from build123d import *

# Parameters (mm, degrees)
F1_DEPTH = 25
F0_R     = 250
F2_DEPTH = 20
F0_R_2   = 130
F3_DEPTH = 15


with BuildPart() as f1:
    # F0 (on Front) → F1 (new body)
    with BuildSketch(Plane.XZ):
        with BuildLine():
            ThreePointArc((79.802773, 564.385965), (0, 490), (-79.802773, 564.385965))
            ThreePointArc((-79.802773, 564.385965), (-570, 0), (-79.802773, -564.385965))
            ThreePointArc((-79.802773, -564.385965), (0, -490), (79.802773, -564.385965))
            ThreePointArc((79.802773, -564.385965), (570, 0), (79.802773, 564.385965))
        make_face()
        with BuildLine():
            ThreePointArc((-330.670307, 225.071429), (-335.875721, 335.875721), (-225.071429, 330.670307))
            ThreePointArc((-225.071429, 330.670307), (0, 400), (225.071429, 330.670307))
            ThreePointArc((225.071429, 330.670307), (308.260755, 353.404197), (357.842712, 282.842712))
            ThreePointArc((357.842712, 282.842712), (350.710487, 250.921478), (330.670307, 225.071429))
            ThreePointArc((330.670307, 225.071429), (400, 0), (330.670307, -225.071429))
            ThreePointArc((330.670307, -225.071429), (350.710487, -250.921478), (357.842712, -282.842712))
            ThreePointArc((357.842712, -282.842712), (308.260755, -353.404197), (225.071429, -330.670307))
            ThreePointArc((225.071429, -330.670307), (0, -400), (-225.071429, -330.670307))
            ThreePointArc((-225.071429, -330.670307), (-335.875721, -335.875721), (-330.670307, -225.071429))
            ThreePointArc((-330.670307, -225.071429), (-400, 0), (-330.670307, 225.071429))
        make_face(mode=Mode.SUBTRACT)
    extrude(amount=F1_DEPTH)

    # F0 (on Front) → F2 (join)
    with BuildSketch(Plane.XZ):
        with BuildLine():
            ThreePointArc((-225.071429, 330.670307), (-212.281228, 308.260755), (-207.842712, 282.842712))
            ThreePointArc((-207.842712, 282.842712), (-250.921478, 214.974938), (-330.670307, 225.071429))
            ThreePointArc((-330.670307, 225.071429), (-400, 0), (-330.670307, -225.071429))
            ThreePointArc((-330.670307, -225.071429), (-250.921478, -214.974938), (-207.842712, -282.842712))
            ThreePointArc((-207.842712, -282.842712), (-212.281228, -308.260755), (-225.071429, -330.670307))
            ThreePointArc((-225.071429, -330.670307), (0, -400), (225.071429, -330.670307))
            ThreePointArc((225.071429, -330.670307), (229.809704, -229.809704), (330.670307, -225.071429))
            ThreePointArc((330.670307, -225.071429), (400, 0), (330.670307, 225.071429))
            ThreePointArc((330.670307, 225.071429), (229.809704, 229.809704), (225.071429, 330.670307))
            ThreePointArc((225.071429, 330.670307), (0, 400), (-225.071429, 330.670307))
        make_face()
        Circle(F0_R, mode=Mode.SUBTRACT)
    extrude(amount=F2_DEPTH)

    # F0 (on Front) → F3 (join)
    with BuildSketch(Plane.XZ):
        Circle(F0_R)
        Circle(F0_R_2, mode=Mode.SUBTRACT)
    extrude(amount=F3_DEPTH)


solid = f1.part
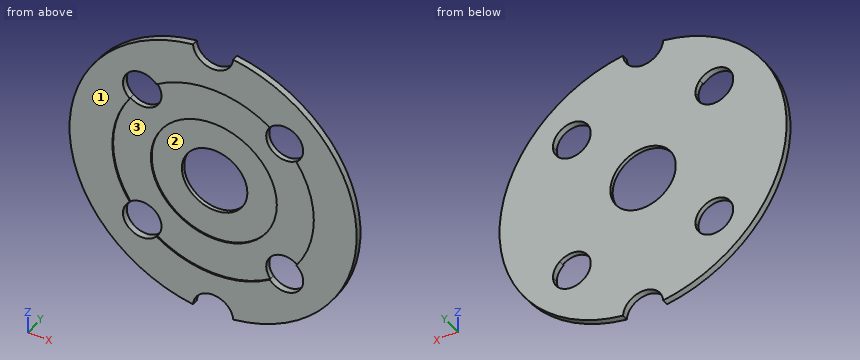
Build history of the part. All positions in model axes, mm. Face numbers are marked on the shaded views. Round coordinates to 2 decimals unless told otherwise and drop trailing zeros. Write each loop counter-clockwise with the first axis right and the second up, starting at its lowest first coordinate (ties: lowest second). Pieces come first, ordered by that corner, then holes. Notation, with made-up numbers: (31.5, 55.25) -> (37.5, 55.25) arc R33 ccw to (37.5, 88.25) -> close; hole circle Ø2 at (16.25, -2). An arc over 180 degrees is marked (long way). Use one line per item in the form item = value.
Q1. Drop flat-ended pins along their axis: P1, Ø1, axis at x = 405.5, y = -18.5, coming from the -Z side; P2, Ø8, axis at x = 175.5, z = 79, coming from the -Y side; P3, Ø2, axis at x = -321, y = -20.5, coming from the -Z side. Give the stop position or say it passes through.
Conclusion:
P1 = -401.09
P2 = -15
P3 = -471.7
Q2. Band-saw the part on B-B, the plane x = 313. Write the cut outline in (y, z).
Conclusion:
outline = (-25, -476.37) -> (0, -476.37) -> (0, -351.51) -> (-25, -351.51) -> close; (-25, 351.51) -> (0, 351.51) -> (0, 476.37) -> (-25, 476.37) -> close; (-20, -214.17) -> (0, -214.17) -> (0, 214.17) -> (-20, 214.17) -> close
Q3. Band-saw the part on D-D, the plane x = 101. Write the cut outline in (y, z).
Conclusion:
outline = (-25, -560.98) -> (0, -560.98) -> (0, -81.85) -> (-15, -81.85) -> (-15, -228.69) -> (-20, -228.69) -> (-20, -387.04) -> (-25, -387.04) -> close; (-25, 387.04) -> (-20, 387.04) -> (-20, 228.69) -> (-15, 228.69) -> (-15, 81.85) -> (0, 81.85) -> (0, 560.98) -> (-25, 560.98) -> close
Q4. Band-saw the part on C-C, the plane y = -5. Write the cut outline in (x, z), then the cut area to 3 significant figures.
Conclusion:
outline = (-79.8, -564.39) arc R80 cw to (79.8, -564.39) arc R570 ccw to (79.8, 564.39) arc R80 cw to (-79.8, 564.39) arc R570 ccw to start; hole (-225.07, -330.67) arc R75 ccw to (-207.84, -282.84) arc R75 ccw (long way) to start; hole (-225.07, 330.67) arc R75 ccw (long way) to (-207.84, 282.84) arc R75 ccw to start; hole circle Ø260 at (0, 0); hole (330.67, -225.07) arc R75 ccw (long way) to (357.84, -282.84) arc R75 ccw to start; hole (330.67, 225.07) arc R75 ccw to (357.84, 282.84) arc R75 ccw (long way) to start
area = 877,000 mm²
Q5. Band-saw the part on A-A, the plane z = 0. Write the cut outline in (x, y), then the cut area to 3 significant figures.
Conclusion:
outline = (-570, -25) -> (-400, -25) -> (-400, -20) -> (-250, -20) -> (-250, -15) -> (-130, -15) -> (-130, 0) -> (-570, 0) -> close; (130, -15) -> (250, -15) -> (250, -20) -> (400, -20) -> (400, -25) -> (570, -25) -> (570, 0) -> (130, 0) -> close
area = 18,100 mm²
Q6. Two-plate mould, pull along Z, no slides. Class the marked faces 1, 2 and 3: released by +Z, released by -Z, zero draft, split by the parting line, or undercut.
Conclusion:
face_1 = zero draft
face_2 = undercut
face_3 = undercut
Q7. Drill centre lines: L1, parallel to Z at x = 0, y = -17.75; L2, parallel to Y at x = -393, z = 55; L3, parallel to Y at x = -84, z = 231. Where is each one in solid material? Low to high.
Conclusion:
L1 = -490 to -250, 250 to 490
L2 = -20 to 0
L3 = -15 to 0
